```python
from build123d import *

# Parameters (mm, degrees)
ESBO_O1_W                = 84
ESBO_O1_H                = 3
RESSALTO_EXTRUS_O1_DEPTH = 194
CORTE_EXTRUS_O1_DEPTH    = 194
CORTE_EXTRUS_O5_DEPTH    = 10
CORTE_EXTRUS_O6_DEPTH    = 10
ESBO_O9_W                = 3.064404225
ESBO_O9_H                = 50.6
RESSALTO_EXTRUS_O2_DEPTH = 3
ESBO_O12_R               = 3
CORTE_EXTRUS_O8_DEPTH    = 3
ESBO_O14_R               = 3
RESSALTO_EXTRUS_O3_DEPTH = 3
ESBO_O16_R               = 3
CORTE_EXTRUS_O9_DEPTH    = 3
ESBO_O17_W               = 1
ESBO_O17_H               = 6.5
CORTE_EXTRUS_O10_DEPTH   = 10
ESBO_O18_W               = 2
ESBO_O18_H               = 6.5
CORTE_EXTRUS_O11_DEPTH   = 10
ESBO_O19_R               = 1.6
CORTE_EXTRUS_O12_DEPTH   = 10
CORTE_EXTRUS_O13_DEPTH   = 10
CORTE_EXTRUS_O14_DEPTH   = 10


with BuildPart() as part:
    # Esboço1 → Ressalto-extrusão1 (new body)
    with BuildSketch(Plane.XY):
        with Locations((-3.22930454, -1.5)):
            Rectangle(ESBO_O1_W, ESBO_O1_H)
    extrude(amount=RESSALTO_EXTRUS_O1_DEPTH)

    # Esboço2 → Corte-extrusão1 (cut)
    with BuildSketch(Plane(origin=(0, 0, 0), x_dir=(1, 0, 0), z_dir=(0, 1, 0))):
        Polygon((-3.22930454, 0), (9.27069546, 0), (9.27069546, -50.6), (-15.72930454, -50.6), (-15.72930454, 0), align=None)
        Polygon((-3.22930454, -194), (9.27069546, -194), (9.27069546, -143.4), (-15.72930454, -143.4), (-15.72930454, -194), align=None)
    extrude(amount=-CORTE_EXTRUS_O1_DEPTH, mode=Mode.SUBTRACT)

    # Esboço7 → Corte-extrusão5 (cut)
    with BuildSketch(Plane(origin=(0, 0, 0), x_dir=(1, 0, 0), z_dir=(0, 1, 0))):
        Polygon((-20.72930454, -50.6), (-3.22930454, -50.6), (14.27069546, -50.6), (14.27069546, 0), (-20.72930454, 0), align=None)
    extrude(amount=-CORTE_EXTRUS_O5_DEPTH, mode=Mode.SUBTRACT)

    # Esboço8 → Corte-extrusão6 (cut)
    with BuildSketch(Plane(origin=(0, 0, 0), x_dir=(1, 0, 0), z_dir=(0, 1, 0))):
        Polygon((14.27069546, -143.4), (-3.22930454, -143.4), (-20.72930454, -143.4), (-20.72930454, -194), (14.27069546, -194), align=None)
    extrude(amount=-CORTE_EXTRUS_O6_DEPTH, mode=Mode.SUBTRACT)

    # Esboço9 → Ressalto-extrusão2 (add)
    with BuildSketch(Plane(origin=(0, 0, 0), x_dir=(1, 0, 0), z_dir=(0, 1, 0))):
        with Locations((-19.197102427, -25.3)):
            Rectangle(ESBO_O9_W, ESBO_O9_H)
        with Locations((12.738493348, -25.3)):
            Rectangle(ESBO_O9_W, ESBO_O9_H)
    extrude(amount=-RESSALTO_EXTRUS_O2_DEPTH)

    # Esboço12 → Corte-extrusão8 (cut)
    with BuildSketch(Plane(origin=(0, 0, 0), x_dir=(1, 0, 0), z_dir=(0, 1, 0))):
        with Locations(Location((22.49182576, -37.95, 0), (0, 0, 270))):
            Circle(ESBO_O12_R)
        with Locations(Location((22.49182576, -25.3, 0), (0, 0, 270))):
            Circle(ESBO_O12_R)
        with Locations(Location((22.49182576, -12.65, 0), (0, 0, 270))):
            Circle(ESBO_O12_R)
        with Locations(Location((-28.94930454, -12.65, 0), (0, 0, 270))):
            Circle(ESBO_O12_R)
        with Locations(Location((-28.94930454, -25.3, 0), (0, 0, 270))):
            Circle(ESBO_O12_R)
        with Locations(Location((-28.94930454, -37.95, 0), (0, 0, 270))):
            Circle(ESBO_O12_R)
    extrude(amount=-CORTE_EXTRUS_O8_DEPTH, mode=Mode.SUBTRACT)

    # Esboço14 → Ressalto-extrusão3 (add)
    with BuildSketch(Plane(origin=(0, 0, 0), x_dir=(1, 0, 0), z_dir=(0, 1, 0))):
        Polygon((38.77069546, -194), (38.77069546, -97), (-45.22930454, -97), (-45.22930454, -194), (-17.664900315, -194), (-17.664900315, -143.4), (11.206291235, -143.4), (11.206291235, -194), align=None)
        with Locations((-28.94930454, -181.35)):
            Circle(ESBO_O14_R, mode=Mode.SUBTRACT)
        with Locations((-28.94930454, -168.7)):
            Circle(ESBO_O14_R, mode=Mode.SUBTRACT)
        with Locations((-28.94930454, -156.05)):
            Circle(ESBO_O14_R, mode=Mode.SUBTRACT)
        with Locations((22.49182576, -181.35)):
            Circle(ESBO_O14_R, mode=Mode.SUBTRACT)
        with Locations((22.49182576, -168.7)):
            Circle(ESBO_O14_R, mode=Mode.SUBTRACT)
        with Locations((22.49182576, -156.05)):
            Circle(ESBO_O14_R, mode=Mode.SUBTRACT)
    extrude(amount=-RESSALTO_EXTRUS_O3_DEPTH)

    # Esboço16 → Corte-extrusão9 (cut)
    with BuildSketch(Plane(origin=(0, 0, 0), x_dir=(1, 0, 0), z_dir=(0, 1, 0))):
        with Locations(Location((22.49182576, -37.95, 0), (0, 0, 270))):
            Circle(ESBO_O16_R)
        with Locations(Location((22.49182576, -25.3, 0), (0, 0, 270))):
            Circle(ESBO_O16_R)
        with Locations(Location((22.49182576, -12.65, 0), (0, 0, 270))):
            Circle(ESBO_O16_R)
        with Locations(Location((-28.94930454, -12.65, 0), (0, 0, 270))):
            Circle(ESBO_O16_R)
        with Locations(Location((-28.94930454, -25.3, 0), (0, 0, 270))):
            Circle(ESBO_O16_R)
        with Locations(Location((-28.94930454, -37.95, 0), (0, 0, 270))):
            Circle(ESBO_O16_R)
        with Locations(Location((-28.94930454, -156.05, 0), (0, 0, 90))):
            Circle(ESBO_O16_R)
        with Locations(Location((-28.94930454, -168.7, 0), (0, 0, 90))):
            Circle(ESBO_O16_R)
        with Locations(Location((-28.94930454, -181.35, 0), (0, 0, 90))):
            Circle(ESBO_O16_R)
        with Locations(Location((22.49182576, -181.35, 0), (0, 0, 90))):
            Circle(ESBO_O16_R)
        with Locations(Location((22.49182576, -168.7, 0), (0, 0, 90))):
            Circle(ESBO_O16_R)
        with Locations(Location((22.49182576, -156.05, 0), (0, 0, 90))):
            Circle(ESBO_O16_R)
    extrude(amount=-CORTE_EXTRUS_O9_DEPTH, mode=Mode.SUBTRACT)

    # Esboço17 → Corte-extrusão10 (cut)
    with BuildSketch(Plane(origin=(0, 0, 0), x_dir=(1, 0, 0), z_dir=(0, 1, 0))):
        with Locations((6.17069546, -53.85)):
            Rectangle(ESBO_O17_W, ESBO_O17_H)
        with Locations((5.17069546, -53.85)):
            Rectangle(ESBO_O17_W, ESBO_O17_H)
        Polygon((-11.12930454, -57.1), (-11.12930454, -50.6), (-12.12930454, -50.6), (-13.12930454, -50.6), (-13.12930454, -57.1), align=None)
    extrude(amount=-CORTE_EXTRUS_O10_DEPTH, mode=Mode.SUBTRACT)

    # Esboço18 → Corte-extrusão11 (cut)
    with BuildSketch(Plane(origin=(0, 0, 0), x_dir=(1, 0, 0), z_dir=(0, 1, 0))):
        with Locations((5.67069546, -140.15)):
            Rectangle(ESBO_O18_W, ESBO_O18_H)
        with Locations((-12.12930454, -140.15)):
            Rectangle(ESBO_O18_W, ESBO_O18_H)
    extrude(amount=-CORTE_EXTRUS_O11_DEPTH, mode=Mode.SUBTRACT)

    # Esboço19 → Corte-extrusão12 (cut)
    with BuildSketch(Plane(origin=(0, 0, 0), x_dir=(1, 0, 0), z_dir=(0, 1, 0))):
        with Locations(Location((-27.22930454, -116, 0), (0, 0, 270))):
            Circle(ESBO_O19_R)
        with Locations(Location((16.27069546, -65.5, 0), (0, 0, 270))):
            Circle(ESBO_O19_R)
        with Locations(Location((-11.72930454, -65.5, 0), (0, 0, 270))):
            Circle(ESBO_O19_R)
    extrude(amount=-CORTE_EXTRUS_O12_DEPTH, mode=Mode.SUBTRACT)

    # Esboço20 → Corte-extrusão13 (cut)
    with BuildSketch(Plane(origin=(0, 0, 0), x_dir=(1, 0, 0), z_dir=(0, 1, 0))):
        Polygon((-3.22930454, -140.6), (1.02069546, -140.6), (1.02069546, -143.4), (-7.47930454, -143.4), (-7.47930454, -140.6), align=None)
    extrude(amount=-CORTE_EXTRUS_O13_DEPTH, mode=Mode.SUBTRACT)

    # Esboço21 → Corte-extrusão14 (cut)
    with BuildSketch(Plane(origin=(0, 0, 0), x_dir=(1, 0, 0), z_dir=(0, 1, 0))):
        Polygon((-3.22930454, -53.4), (-7.47930454, -53.4), (-7.47930454, -50.6), (1.02069546, -50.6), (1.02069546, -53.4), align=None)
    extrude(amount=-CORTE_EXTRUS_O14_DEPTH, mode=Mode.SUBTRACT)


solid = part.part
```
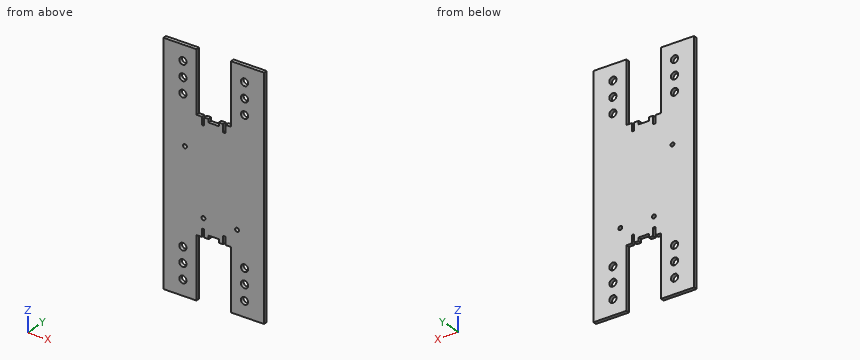
CAD build for the part. Positions are in the model's coordinates, mm. Give positions to 0.01 mm unless a question says otherwise; leave off trailing zeros. Write each loop counter-clockwise with the first axis right and the second up, starting at its lowest first coordinate (ties: lowest second). Pieces come first, ordered by that corner, then holes. Notation, with made-up numbers: M 39.5,11 L 86.5,11 A24 ccw 86.5,21 Z; hole C -34.75,67.25 d2. An arc over 180 degrees is marked long. Return JSON: item names as keys, results as strings. Group by question number.
(1) Drill centre lines: L1, parallel to X at y = -1.3, z = 37.95; L2, parallel to X at y = -1.25, z = 181.5; L3, parallel to X at y = -0.65, z = 47. Where is each one in solid material? Low to high. Write a range as [from, to].
(2) Flat gauge pins, fed straight in: pin 1 Ø0.9 at (x, y) = (-16, -1.5) entering from +Z; pin 2 Ø0.9 at (x, y) = (-9, -2) entering from -Z. Where does each tip first touch, or does it go through?
(3) Band-saw the part on B-B (z = 12.65). Give the cut face in (x, y), and give its area (3 significant figures).
(4) Band-saw the part on C-C (y = -1.85). State how many separate pieces and enclosed holes the cut face has, and give its area (3 significant figures).
(5) Band-saw the part on A-A (z = 174). Give the cut face in (x, y).
Entries:
{
 "1": {"L1": "x = [-45.23, -31.95], [-25.95, -17.66], [11.21, 19.49], [25.49, 38.77]", "L2": "x = [-45.23, -31.95], [-25.95, -17.66], [11.21, 19.5], [25.49, 38.77]", "L3": "x = [-45.23, -17.66], [11.21, 38.77]"},
 "2": {"pin 1": "stops at z = 143.4", "pin 2": "stops at z = 50.6"},
 "3": {"outline": "M -45.23,-3 L -31.95,-3 L -31.95,0 L -45.23,0 Z; M -25.95,-3 L -17.66,-3 L -17.66,0 L -25.95,0 Z; M 11.21,-3 L 19.49,-3 L 19.49,0 L 11.21,0 Z; M 25.49,-3 L 38.77,-3 L 38.77,0 L 25.49,0 Z", "area": "129 mm^2"},
 "4": {"separate pieces": "1", "enclosed holes": "15", "area": "12,900 mm^2"},
 "5": {"outline": "M -45.23,-3 L -17.66,-3 L -17.66,0 L -45.23,0 Z; M 11.21,-3 L 38.77,-3 L 38.77,0 L 11.21,0 Z"}
}
